Design review of the part built by this model. Coordinates are the model's own, in mm. Round coordinates to 2 decimals unless told otherwise and drop trailing zeros. Order: outer loops, then holes, each group sorted by start corner. A loop starts at its lowest first (then second) coordinate and runs counter-clockwise, first axis right, second up.
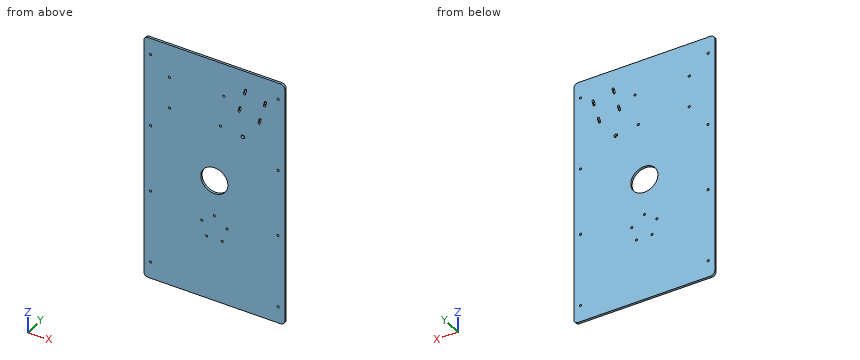
from build123d import *

# Parameters (mm, degrees)
BOSS_EXTRUDE1_DEPTH     = 3.302
M3_CLEARANCE_HOLE1_D    = 3.4
SKETCH6_W               = 210.566
SKETCH6_H               = 3.302
BOSS_EXTRUDE3_DEPTH     = 1.62
SKETCH7_W               = 210.566
SKETCH7_H               = 3.302
BOSS_EXTRUDE4_DEPTH     = 5.18
M3_CLEARANCE_HOLE2_D    = 3.4
SKETCH21_R              = 20.32
CUT_EXTRUDE1_DEPTH      = 336.371396057
ADVANCEDHOLE1_OUTLINE_R = 1.6
ADVANCEDHOLE1_DEPTH     = 3.302
CUT_EXTRUDE2_REACH      = 337.371
SKETCH33_W              = 167.386
SKETCH33_H              = 21.59
FILLET1_R               = 6.35
CUT_EXTRUDE3_DEPTH      = 315.946962825
M5_CLEARANCE_HOLE1_D    = 5.5
M3_CLEARANCE_HOLE3_D    = 3.4


# Read off the part's stored shape, not the designer's step: AdvancedHole1
with BuildPart() as part:
    # Sketch1 → Boss-Extrude1 (new body)
    with BuildSketch(Plane(origin=(0, 0, 0), x_dir=(1, 0, 0), z_dir=(0, 1, 0))):
        Polygon((105.283, -80.01), (105.283, 101.6), (-105.283, 101.6), (-105.283, -80.01), (-83.693, -80.01), (-83.693, -101.6), (83.693, -101.6), (83.693, -80.01), align=None)
    extrude(amount=BOSS_EXTRUDE1_DEPTH)

    # M3 Clearance Hole1 (through all)
    with Locations(Plane(origin=(0, 3.302, 0), x_dir=(1, 0, 0), z_dir=(0, 1, 0))):
        with Locations((-95.377, -54.61), (-95.377, 57.15), (95.377, 57.15), (95.377, -54.61)):
            Hole(M3_CLEARANCE_HOLE1_D / 2)

    # Sketch6 → Boss-Extrude3 (add)
    with BuildSketch(Plane(origin=(0, 0, -101.6), x_dir=(-1, 0, 0), z_dir=(0, 0, -1))):
        with Locations((0, 1.651)):
            Rectangle(SKETCH6_W, SKETCH6_H)
    extrude(amount=BOSS_EXTRUDE3_DEPTH)

    # Sketch7 → Boss-Extrude4 (add)
    with BuildSketch(Plane(origin=(0, 0, -103.22), x_dir=(-1, 0, 0), z_dir=(0, 0, -1))):
        with Locations((0, 1.651)):
            Rectangle(SKETCH7_W, SKETCH7_H)
    extrude(amount=BOSS_EXTRUDE4_DEPTH)


with BuildPart() as body_2:
    # Mirror2: mirrored copy
    add(part.part.mirror(Plane(origin=(0, 0, -108.4), x_dir=(1, 0, 0), z_dir=(0, 0, -1))))


with BuildPart() as part_1:
    add(part.part)

    # Combine1: union body 2
    add(body_2.part)

    # M3 Clearance Hole2 (through all)
    with Locations(Plane(origin=(0, 3.302, 0), x_dir=(1, 0, 0), z_dir=(0, 1, 0))):
        with Locations((-58.293, -91.6), (58.293, -91.6), (-58.293, 308.4), (58.293, 308.4)):
            Hole(M3_CLEARANCE_HOLE2_D / 2)

    # Sketch21 → Cut-Extrude1 (cut, through all)
    with BuildSketch(Plane(origin=(0, 3.302, 0), x_dir=(1, 0, 0), z_dir=(0, 1, 0))):
        with Locations(Location((0, 108.4, 0), (0, 0, 270))):
            Circle(SKETCH21_R)
    extrude(amount=-CUT_EXTRUDE1_DEPTH, mode=Mode.SUBTRACT)

    # AdvancedHole1 outline → AdvancedHole1 (cut)
    with BuildSketch(Plane(origin=(0, 0, 0), x_dir=(1, 0, 0), z_dir=(0, 1, 0))):
        with Locations((-11.624680448, 199.4)):
            Circle(ADVANCEDHOLE1_OUTLINE_R)
        with Locations((-18.809128073, 177.28854382)):
            Circle(ADVANCEDHOLE1_OUTLINE_R)
        with Locations((0, 163.62291236)):
            Circle(ADVANCEDHOLE1_OUTLINE_R)
        with Locations((18.809128073, 177.28854382)):
            Circle(ADVANCEDHOLE1_OUTLINE_R)
        with Locations((11.624680448, 199.4)):
            Circle(ADVANCEDHOLE1_OUTLINE_R)
    extrude(amount=ADVANCEDHOLE1_DEPTH, mode=Mode.SUBTRACT)

    # Sketch33 → Cut-Extrude2 (cut, up to next)
    with BuildSketch(Plane(origin=(0, 3.302, 0), x_dir=(1, 0, 0), z_dir=(0, 1, 0)), mode=Mode.PRIVATE) as cut_extrude2_sk1:
        with Locations((0, 307.605)):
            Rectangle(SKETCH33_W, SKETCH33_H)
    cut_extrude2_tool1 = extrude(cut_extrude2_sk1.sketch, amount=-CUT_EXTRUDE2_REACH, mode=Mode.PRIVATE) & part_1.part
    # Sketch33 → Cut-Extrude2 (cut, up to next)
    with BuildSketch(Plane(origin=(0, 3.302, 0), x_dir=(1, 0, 0), z_dir=(0, 1, 0)), mode=Mode.PRIVATE) as cut_extrude2_sk2:
        with Locations((0, -90.805)):
            Rectangle(SKETCH33_W, SKETCH33_H)
    cut_extrude2_tool2 = extrude(cut_extrude2_sk2.sketch, amount=-CUT_EXTRUDE2_REACH, mode=Mode.PRIVATE) & part_1.part
    add(cut_extrude2_tool1.solids().sort_by_distance((0, 3.302, -307.605))[0], mode=Mode.SUBTRACT)
    add(cut_extrude2_tool2.solids().sort_by_distance((0, 3.302, 90.805))[0], mode=Mode.SUBTRACT)

    # Fillet1
    fillet1_edges = [part_1.edges().sort_by_distance(p)[0] for p in [
        (-105.283, 1.651, 80.01),
        (105.283, 1.651, 80.01),
        (105.283, 1.651, -296.81),
        (-105.283, 1.651, -296.81),
    ]]
    fillet(fillet1_edges, radius=FILLET1_R)

    # Sketch24 → Cut-Extrude3 (cut, through all)
    with BuildSketch(Plane(origin=(0, 3.302, 0), x_dir=(1, 0, 0), z_dir=(0, 1, 0))):
        with BuildLine():
            Line((68.288075685, -5.771611822), (70.099809001, -12.533092606))
            ThreePointArc((70.099809001, -12.533092606), (69.039148829, -14.370209913), (67.202031522, -13.309549741))
            Line((67.202031522, -13.309549741), (65.390298207, -6.548068957))
            ThreePointArc((65.390298207, -6.548068957), (66.450958378, -4.71095165), (68.288075685, -5.771611822))
        make_face()
        with BuildLine():
            Line((76.311466084, -35.715312437), (78.123199399, -42.476793221))
            ThreePointArc((78.123199399, -42.476793221), (77.062539228, -44.313910528), (75.22542192, -43.253250356))
            Line((75.22542192, -43.253250356), (73.413688605, -36.491769572))
            ThreePointArc((73.413688605, -36.491769572), (74.474348777, -34.654652265), (76.311466084, -35.715312437))
        make_face()
        with BuildLine():
            Line((38.34437507, -13.79500222), (40.156108386, -20.556483004))
            ThreePointArc((40.156108386, -20.556483004), (39.095448214, -22.393600311), (37.258330907, -21.332940139))
            Line((37.258330907, -21.332940139), (35.446597592, -14.571459355))
            ThreePointArc((35.446597592, -14.571459355), (36.507257763, -12.734342048), (38.34437507, -13.79500222))
        make_face()
        with BuildLine():
            Line((46.367765469, -43.738702835), (48.179498784, -50.500183619))
            ThreePointArc((48.179498784, -50.500183619), (47.118838613, -52.337300926), (45.281721306, -51.276640754))
            Line((45.281721306, -51.276640754), (43.46998799, -44.51515997))
            ThreePointArc((43.46998799, -44.51515997), (44.530648162, -42.678042663), (46.367765469, -43.738702835))
        make_face()
    extrude(amount=-CUT_EXTRUDE3_DEPTH, mode=Mode.SUBTRACT)

    # M5 Clearance Hole1 (through all)
    with Locations(Plane(origin=(0, 3.302, 0), x_dir=(1, 0, 0), z_dir=(0, 1, 0))):
        with Locations((42.731024346, 23.92564608)):
            Hole(M5_CLEARANCE_HOLE1_D / 2)

    # M3 Clearance Hole3 (through all)
    with Locations(Plane(origin=(0, 3.302, 0), x_dir=(1, 0, 0), z_dir=(0, 1, 0))):
        with Locations((9.017, 19.05), (14.097, -29.21), (-67.183, 19.05), (-67.183, -29.21)):
            Hole(M3_CLEARANCE_HOLE3_D / 2)


solid = part_1.part
1) To check wall thickness, follow line 1 along X through (y, z) = (0.75, -199.4); line 2 along X through (y, z) = (1, -159.65); line 3 along Z through (x, y) = (-15.5, 1.55). State the ranges of each line that lie inside material, in increasing order.
Results:
line 1: x = -105.28 to -13.22, -10.02 to 10.02, 13.22 to 105.28
line 2: x = -105.28 to -97.08, -93.68 to 93.68, 97.08 to 105.28
line 3: z = -296.81 to -121.54, -95.26 to 80.01
2) Take a section at A-A on z = -108.4. Give the boundary of the cut face in (x, y).
Results:
outline: (-105.28, 0) - (-20.32, 0) - (-20.32, 3.3) - (-105.28, 3.3) - close; (20.32, 0) - (105.28, 0) - (105.28, 3.3) - (20.32, 3.3) - close
3) Take a section at B-B on y = 2.6. State how many separate pieces and enclosed holes the cut face has, plus the area to 3 significant figures.
Results:
separate pieces: 1
enclosed holes: 23
area: 77,700 mm2
